```python
from build123d import *

# Parameters (mm, degrees)
F0_W     = 75
F0_H     = 75
F1_DEPTH = 25
F2_R     = 1
F3_DEPTH = 10
F4_R     = 1
F5_DEPTH = 15


with BuildPart() as f1:
    # F0 (on Front) → F1 (new body)
    with BuildSketch(Plane.XZ):
        Rectangle(F0_W, F0_H)
    extrude(amount=F1_DEPTH)

    # F2 (on face) → F3 (cut)
    with BuildSketch(Plane(origin=(0, 0, 0), x_dir=(-1, 0, 0), z_dir=(0, 1, 0))):
        Circle(F2_R)
    extrude(amount=-F3_DEPTH, mode=Mode.SUBTRACT)

    # F4 (on face) → F5 (join)
    with BuildSketch(Plane(origin=(0, 0, 0), x_dir=(-1, 0, 0), z_dir=(0, 1, 0))):
        with Locations((-12.5, 0)):
            Circle(F4_R)
    extrude(amount=F5_DEPTH)


solid = f1.part
```
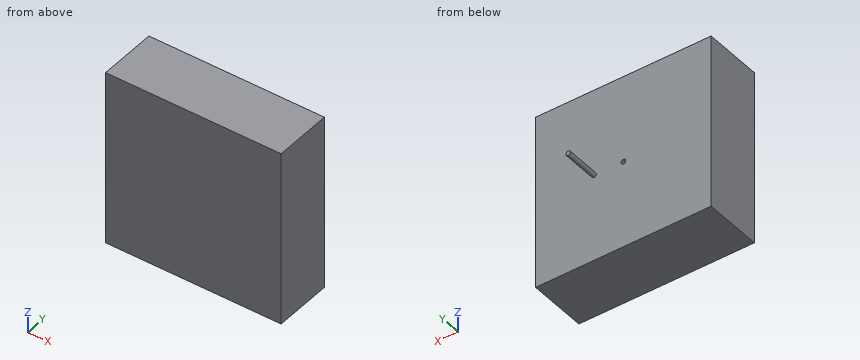
Geometry: final body of the model. Coordinates: model frame, mm. Coordinates: 2 decimals unless noted, no trailing zeros. Order: outer loops, then holes, each group sorted by start corner. A loop starts at its lowest first (then second) coordinate and runs counter-clockwise, first axis right, second up. Notation, with made-up numbers: M 16.5,74.5 L 28.5,74.5 A10 cw 28.5,91.5 Z; hole C -22,35.5 d11. An arc over 180 degrees is marked long. Answer in a Markdown table with one row per item. Add a question column.
Q1. Section query A-A on x = 0. Return the cut outline in (y, z).
Q2. Section query C-C on y = 7.5. Return the cut outline in (x, z), and give its area (3 significant figures).
Q3. Section query B-B on z = 0. Return the cut outline in (x, y), and give its area (4 significant figures).
Q4. Line query: L1, parallel to Z at x = 0, y = -3; L2, parallel to Y at x = -5.5, z = 16.5. Output: solid intervals per line, ascending.
Q5. Section query D-D on x = 12.5. Return the cut outline in (y, z).
Q6. Contact query for flat-ended pins moving along their axis: P1, Ø1.5, axis at x = -17.5, z = 18, coming from the +Y side; P2, Ø1.6, axis at x = 0, z = 0, coming from the +Y side. Output: stop coordinate, or through.
Completed:
| question | item | result |
|---|---|---|
| 1 | outline | M -25,-37.5 L 0,-37.5 L 0,-1 L -10,-1 L -10,1 L 0,1 L 0,37.5 L -25,37.5 Z |
| 2 | outline | C 12.5,0 d2 |
| 2 | area | 3.14 mm2 |
| 3 | outline | M -37.5,-25 L 37.5,-25 L 37.5,0 L 13.5,0 L 13.5,15 L 11.5,15 L 11.5,0 L 1,0 L 1,-10 L -1,-10 L -1,0 L -37.5,0 Z |
| 3 | area | 1,885 mm2 |
| 4 | L1 | z = -37.5 to -1, 1 to 37.5 |
| 4 | L2 | y = -25 to 0 |
| 5 | outline | M -25,-37.5 L 0,-37.5 L 0,-1 L 15,-1 L 15,1 L 0,1 L 0,37.5 L -25,37.5 Z |
| 6 | P1 | stops at y = 0 |
| 6 | P2 | stops at y = -10 |
